Model file for the job. Use its own axes, mm. Face numbers are marked on the shaded views. A direction names the side the tool comes from. Give positions to 0.01 mm unless a question says otherwise; leave off trailing zeros. Write each loop counter-clockwise with the first axis right and the second up, starting at its lowest first coordinate (ties: lowest second). Pieces come first, ordered by that corner, then holes. Notation, with made-up numbers: M -36.5,39 L 18.5,39 A32 ccw 18.5,71 Z; hole C -15,64 d10. An arc over 180 degrees is marked long. Answer as a JSON object with one key per item and string values. Group by question number.
```python
from build123d import *

# Parameters (mm, degrees)
F0_W     = 100
F0_H     = 100
F1_DEPTH = 3
F2_DEPTH = 50
F3_R     = 3


with BuildPart() as f1:
    # F0 (on Top) → F1 (new body)
    with BuildSketch(Plane.XY):
        with Locations((3.506646, -1.476071)):
            Rectangle(F0_W, F0_H)
    extrude(amount=F1_DEPTH)

    # F0 (on Top) → F2 (join)
    with BuildSketch(Plane.XY):
        with BuildLine():
            Line((53.506646, 53.523929), (-46.493354, 53.523929))
            ThreePointArc((-46.493354, 53.523929), (-50.028888, 52.059462), (-51.493354, 48.523929))
            Line((-51.493354, 48.523929), (-51.493354, -51.476071))
            ThreePointArc((-51.493354, -51.476071), (-50.028888, -55.011605), (-46.493354, -56.476071))
            Line((-46.493354, -56.476071), (53.506646, -56.476071))
            ThreePointArc((53.506646, -56.476071), (57.04218, -55.011605), (58.506646, -51.476071))
            Line((58.506646, -51.476071), (58.506646, 48.523929))
            ThreePointArc((58.506646, 48.523929), (57.04218, 52.059462), (53.506646, 53.523929))
        make_face()
        with Locations((3.506646, -1.476071)):
            Rectangle(F0_W, F0_H, mode=Mode.SUBTRACT)
    extrude(amount=F2_DEPTH)

    # F3
    f3_edges = [f1.edges().sort_by_distance(p)[0] for p in [
        (-51.493354, -1.476071, 50),
    ]]
    fillet(f3_edges, radius=F3_R)


solid = f1.part
```
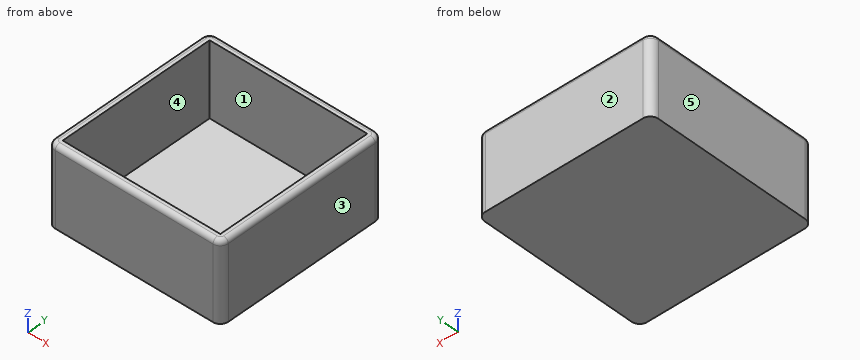
Q1. Wall check: L1, parallel to X at y = 20, z = 12; L2, parallel to Y at x = -5, z = 34.5; L3, parallel to Z at x = 34.5, y = 19. Give the ranges that are in metal, low to high.
Q2. Slice it at C-C, the plane x = 3. Write the cut outline in (y, z).
Q3. Slice it at B-B, the plane y = -5.5. Write the cut outline in (x, z).
Q4. Slice it at A-A, the plane z = 40.5. Write the cut outline in (x, y), then the cut area to 3 significant figures.
Q5. Drop a flat-ended pin along its axis: P1, Ø6, axis at x = -8, y = -18, coming from the +Z side. Give the stop position or say it passes through.
Q6. Two-plate mould, pull along Y, no slides. Class the marked faces 1, 2 and 3: +Y half, -Y half, draft (parallel to the pull), parting line (faces both ways), or undercut.
Q7. 3-axis set-ups, long thin cutter, end or side, ignore diameter. For the marked faces 4 and 5: which of +Z, -Z, +X, -X, +Y, -Y reach the whole face in a straight line?
Solved:
{
 "1": {"L1": "x = -51.49 to -46.49, 53.51 to 58.51", "L2": "y = -56.48 to -51.48, 48.52 to 53.52", "L3": "z = 0 to 3"},
 "2": {"outline": "M -56.48,0 L 53.52,0 L 53.52,47 A3 ccw 50.52,50 L 48.52,50 L 48.52,3 L -51.48,3 L -51.48,50 L -53.48,50 A3 ccw -56.48,47 Z"},
 "3": {"outline": "M -51.49,0 L 58.51,0 L 58.51,47 A3 ccw 55.51,50 L 53.51,50 L 53.51,3 L -46.49,3 L -46.49,50 L -48.49,50 A3 ccw -51.49,47 Z"},
 "4": {"outline": "M -51.49,-51.48 A5 ccw -46.49,-56.48 L 53.51,-56.48 A5 ccw 58.51,-51.48 L 58.51,48.52 A5 ccw 53.51,53.52 L -46.49,53.52 A5 ccw -51.49,48.52 Z; hole M -46.49,-51.48 L 53.51,-51.48 L 53.51,48.52 L -46.49,48.52 Z", "area": "2,080 mm²"},
 "5": {"P1": "stops at z = 3"},
 "6": {"face 1": "undercut", "face 2": "+Y half", "face 3": "draft"},
 "7": {"face 4": "+Z", "face 5": "+Z, -Z, -X, +Y, -Y"}
}
